```python
from build123d import *

# Parameters (mm, degrees)
CROQUIS1_R                   = 2.5
SALIENTE_EXTRUIR1_DEPTH      = 5
SALIENTE_EXTRUIR2_DEPTH      = 6
SALIENTE_EXTRUIR5_DEPTH      = 2
SALIENTE_EXTRUIR5_DEPTH_BACK = 0.1
CROQUIS2_W                   = 41.5
CROQUIS2_H                   = 5.75
CROQUIS2_H_2                 = 4
CROQUIS2_H_3                 = 1.75
CROQUIS2_W_2                 = 1.75
CROQUIS3_R                   = 2
SALIENTE_EXTRUIR6_DEPTH      = 8
CORTAR_EXTRUIR1_REACH        = 36.373
CORTAR_EXTRUIR2_START        = -3
CROQUIS4_R                   = 3.5
CROQUIS4_R_2                 = 2
CORTAR_EXTRUIR2_DEPTH        = 3
REDONDEO1_R                  = 2
REDONDEO2_R                  = 2


with BuildPart() as part:
    # Croquis1 → Saliente-Extruir1 (new body)
    with BuildSketch(Plane(origin=(0, 0, 0), x_dir=(1, 0, 0), z_dir=(0, 1, 0))):
        with BuildLine():
            Line((-22.5, -22.5), (22.5, -22.5))
            Line((22.5, -22.5), (22.5, -20.75))
            Line((22.5, -20.75), (-3.5, -20.75))
            ThreePointArc((-3.5, -20.75), (-7.5, -16.75), (-3.5, -12.75))
            Line((-3.5, -12.75), (22.5, -12.75))
            Line((22.5, -12.75), (22.5, 22.5))
            Line((22.5, 22.5), (-22.5, 22.5))
            Line((-22.5, 22.5), (-22.5, 20.75))
            Line((-22.5, 20.75), (3.5, 20.75))
            ThreePointArc((3.5, 20.75), (7.5, 16.75), (3.5, 12.75))
            Line((3.5, 12.75), (-22.5, 12.75))
            Line((-22.5, 12.75), (-22.5, -22.5))
        make_face()
        with Locations(Location((0, 0, 0), (0, 0, 270))):
            Circle(CROQUIS1_R, mode=Mode.SUBTRACT)
    extrude(amount=-SALIENTE_EXTRUIR1_DEPTH)

    # Croquis1<3> → Saliente-Extruir2 (add)
    with BuildSketch(Plane(origin=(0, 0, 0), x_dir=(1, 0, 0), z_dir=(0, 1, 0))):
        Polygon((-22.5, 7.75), (-22.5, -22.5), (22.5, -22.5), (22.5, -20.75), (-3.5, -20.75), (-20.75, -20.75), (-20.75, 7.75), align=None)
        Polygon((-22.5, 22.5), (-22.5, 20.75), (3.5, 20.75), (20.75, 20.75), (20.75, -7.75), (22.5, -7.75), (22.5, 22.5), align=None)
    extrude(amount=SALIENTE_EXTRUIR2_DEPTH)

    # Croquis2 → Saliente-Extruir5 (add, two sides: drawn at the far end of the back side and taken through both)
    with BuildSketch(Plane(origin=(0, 6, 0), x_dir=(1, 0, 0), z_dir=(0, 1, 0)).offset(-SALIENTE_EXTRUIR5_DEPTH_BACK)):
        with Locations((0, 19.625)):
            Rectangle(CROQUIS2_W, CROQUIS2_H)
        Polygon((-20.75, 22.5), (-22.5, 22.5), (-22.5, 7.75), (-20.75, 7.75), (-20.75, 16.75), align=None)
        with Locations((0, -18.75)):
            Rectangle(CROQUIS2_W, CROQUIS2_H_2)
        with Locations((0, -21.625)):
            Rectangle(CROQUIS2_W, CROQUIS2_H_3)
        Polygon((-20.75, 7.75), (-22.5, 7.75), (-22.5, -22.5), (-20.75, -22.5), (-20.75, -20.75), (-20.75, -16.75), align=None)
        Polygon((22.5, 22.5), (20.75, 22.5), (20.75, 16.75), (20.75, -16.75), (20.75, -20.75), (22.5, -20.75), align=None)
        with Locations((21.625, -21.625)):
            Rectangle(CROQUIS2_W_2, CROQUIS2_H_3)
    extrude(amount=SALIENTE_EXTRUIR5_DEPTH + SALIENTE_EXTRUIR5_DEPTH_BACK)

    # Croquis3 → Saliente-Extruir6 (add)
    with BuildSketch(Plane(origin=(0, 8, 0), x_dir=(1, 0, 0), z_dir=(0, 1, 0))):
        with BuildLine():
            Line((-20.75, 5), (-20.75, -5))
            Line((-20.75, -5), (-17.5, -5))
            Line((-17.5, -5), (-17.5, -2))
            ThreePointArc((-17.5, -2), (-19.5, 0), (-17.5, 2))
            Line((-17.5, 2), (-17.5, 5))
            Line((-17.5, 5), (-20.75, 5))
        make_face()
        with Locations((-17.5, 0)):
            Circle(CROQUIS3_R)
        with BuildLine():
            Line((-17.5, -5), (-17.5, 5))
            ThreePointArc((-17.5, 5), (-12.5, 0), (-17.5, -5))
        make_face()
        with BuildLine():
            ThreePointArc((-17.5, 2), (-19.5, 0), (-17.5, -2))
            Line((-17.5, -2), (-17.5, 2))
        make_face()
        with BuildLine():
            Line((-17.5, 2), (-17.5, -2))
            ThreePointArc((-17.5, -2), (-16.085786438, -1.414213562), (-15.5, 0))
            ThreePointArc((-15.5, 0), (-16.085786438, 1.414213562), (-17.5, 2))
        make_face()
    saliente_extruir6 = extrude(amount=-SALIENTE_EXTRUIR6_DEPTH)

    # Croquis3<3> → Cortar-Extruir1 (cut, up to next)
    with BuildSketch(Plane(origin=(0, 8, 0), x_dir=(1, 0, 0), z_dir=(0, 1, 0)), mode=Mode.PRIVATE) as cortar_extruir1_sk1:
        with BuildLine():
            ThreePointArc((-17.5, 2), (-19.5, 0), (-17.5, -2))
            Line((-17.5, -2), (-17.5, 2))
        make_face()
    cortar_extruir1_tool1 = extrude(cortar_extruir1_sk1.sketch, amount=-CORTAR_EXTRUIR1_REACH, mode=Mode.PRIVATE) & part.part
    # Croquis3<3> → Cortar-Extruir1 (cut, up to next)
    with BuildSketch(Plane(origin=(0, 8, 0), x_dir=(1, 0, 0), z_dir=(0, 1, 0)), mode=Mode.PRIVATE) as cortar_extruir1_sk2:
        with BuildLine():
            Line((-17.5, 2), (-17.5, -2))
            ThreePointArc((-17.5, -2), (-16.085786438, -1.414213562), (-15.5, 0))
            ThreePointArc((-15.5, 0), (-16.085786438, 1.414213562), (-17.5, 2))
        make_face()
    cortar_extruir1_tool2 = extrude(cortar_extruir1_sk2.sketch, amount=-CORTAR_EXTRUIR1_REACH, mode=Mode.PRIVATE) & part.part
    # Croquis3<3> → Cortar-Extruir1 (cut, up to next)
    with BuildSketch(Plane(origin=(0, 8, 0), x_dir=(1, 0, 0), z_dir=(0, 1, 0)), mode=Mode.PRIVATE) as cortar_extruir1_sk3:
        with BuildLine():
            ThreePointArc((-17.5, 2), (-19.5, 0), (-17.5, -2))
            Line((-17.5, -2), (-17.5, 2))
        make_face()
    cortar_extruir1_tool3 = extrude(cortar_extruir1_sk3.sketch, amount=-CORTAR_EXTRUIR1_REACH, mode=Mode.PRIVATE) & part.part
    # Croquis3<3> → Cortar-Extruir1 (cut, up to next)
    with BuildSketch(Plane(origin=(0, 8, 0), x_dir=(1, 0, 0), z_dir=(0, 1, 0)), mode=Mode.PRIVATE) as cortar_extruir1_sk4:
        with BuildLine():
            Line((-17.5, 2), (-17.5, -2))
            ThreePointArc((-17.5, -2), (-16.085786438, -1.414213562), (-15.5, 0))
            ThreePointArc((-15.5, 0), (-16.085786438, 1.414213562), (-17.5, 2))
        make_face()
    cortar_extruir1_tool4 = extrude(cortar_extruir1_sk4.sketch, amount=-CORTAR_EXTRUIR1_REACH, mode=Mode.PRIVATE) & part.part
    cortar_extruir1_1 = cortar_extruir1_tool1.solids().sort_by_distance((-18.348826, 8, 0))[0]
    add(cortar_extruir1_1, mode=Mode.SUBTRACT)
    cortar_extruir1_2 = cortar_extruir1_tool2.solids().sort_by_distance((-16.651174, 8, 0))[0]
    add(cortar_extruir1_2, mode=Mode.SUBTRACT)
    cortar_extruir1_3 = cortar_extruir1_tool3.solids().sort_by_distance((-18.348826, 8, 0))[0]
    add(cortar_extruir1_3, mode=Mode.SUBTRACT)
    cortar_extruir1_4 = cortar_extruir1_tool4.solids().sort_by_distance((-16.651174, 8, 0))[0]
    add(cortar_extruir1_4, mode=Mode.SUBTRACT)
    cortar_extruir1 = cortar_extruir1_1 + cortar_extruir1_2 + cortar_extruir1_3 + cortar_extruir1_4  # Cortar-Extruir1 as one shape, for the pattern or mirror that repeats it

    # Simetría1: Saliente-Extruir6, Cortar-Extruir1 across plane
    add(saliente_extruir6.mirror(Plane(origin=(0, 0, 0), x_dir=(0, 0, 1), z_dir=(1, 0, 0))))
    add(cortar_extruir1.mirror(Plane(origin=(0, 0, 0), x_dir=(0, 0, 1), z_dir=(1, 0, 0))), mode=Mode.SUBTRACT)

    # Croquis4 → Cortar-Extruir2 (cut)
    # profile 1 of 2: a face of its own
    with BuildSketch(Plane.XZ.offset(5).offset(CORTAR_EXTRUIR2_START)):
        with Locations(Location((-17.5, 0, 0), (0, 0, 270))):
            Circle(CROQUIS4_R)
        with Locations(Location((-17.5, 0, 0), (0, 0, 90))):
            Circle(CROQUIS4_R_2, mode=Mode.SUBTRACT)
    # profile 2 of 2: a face of its own
    with BuildSketch(Plane.XZ.offset(5).offset(CORTAR_EXTRUIR2_START)):
        with Locations(Location((17.5, 0, 0), (0, 0, 270))):
            Circle(CROQUIS4_R)
        with Locations(Location((17.5, 0, 0), (0, 0, 90))):
            Circle(CROQUIS4_R_2, mode=Mode.SUBTRACT)
    extrude(amount=CORTAR_EXTRUIR2_DEPTH, mode=Mode.SUBTRACT)

    # Redondeo1
    redondeo1_edges = [part.edges().sort_by_distance(p)[0] for p in [
        (20.75, 6.95, 16.75),
        (-20.75, 6.95, 16.75),
        (20.75, 6.95, -16.75),
        (-20.75, 4, -5),
        (-20.75, 4, 5),
        (20.75, 4, 5),
        (20.75, 4, -5),
        (-20.75, 6.95, -16.75),
    ]]
    fillet(redondeo1_edges, radius=REDONDEO1_R)

    # Redondeo2
    redondeo2_edges = [part.edges().sort_by_distance(p)[0] for p in [
        (-22.5, 1.5, -22.5),
        (22.5, 1.5, -22.5),
        (-22.5, 1.5, 22.5),
        (22.5, 1.5, 22.5),
        (20.75, 2.95, -20.75),
        (-20.75, 2.95, 20.75),
    ]]
    fillet(redondeo2_edges, radius=REDONDEO2_R)


solid = part.part
```
Geometry check sheet. Reference: the model listing, model coordinates, mm. A direction names the side the tool comes from. Round coordinates to 2 decimals unless told otherwise and drop trailing zeros. Loops run counter-clockwise (first coordinate to the right, second up) from the corner with the lowest first, then second, coordinate; pieces in that order, holes last. Notation, with made-up numbers: (0, 57) -> (44, 57) arc R23 cw to (44, 94) -> close; hole circle Ø5 at (88, -23.5). An arc over 180 degrees is marked (long way). Use a Markdown table: item, result.
(1) Mould release check, pull along Z, two halves, no side actions. Record for faces 4 (the flat face through (0, -5, 5)), 5 (the cylindrical face through (7.5, -2.5, -16.8)), 6 (the cylindrical face through (21.9, 1.59, -21.93)): released by +Z, released by -Z, zero draft, split by the parting line, or undercut.
Calculated:
| item | result |
|---|---|
| face 4 | zero draft |
| face 5 | undercut |
| face 6 | released by -Z |
(2) Sectioned sample at C-C (x = -9). Enter the section's corners in (y, z).
Calculated:
| item | result |
|---|---|
| outline | (-5, -22.5) -> (8, -22.5) -> (8, -16.75) -> (5.9, -16.75) -> (5.9, -20.75) -> (-5, -20.75) -> close; (-5, -12.75) -> (0, -12.75) -> (0, 20.75) -> (5.9, 20.75) -> (5.9, 16.75) -> (8, 16.75) -> (8, 22.5) -> (-5, 22.5) -> close |
(3) Go/stop test with flat-tipped pins: P1, Ø6.5, axis at y = 5.5, z = 15.5, coming from the +X side; P2, Ø4, axis at x = -11.5, z = 14.5, coming from the +Y side; P3, Ø0.9, axis at x = -21.5, y = 2.5, coming from the -Z side; P4, Ø1, axis at y = 4.5, z = -15.5, coming from the -X side. Record where each tip stops, or that it passes through.
Calculated:
| item | result |
|---|---|
| P1 | x = 22.5 |
| P2 | y = 0 |
| P3 | z = -22.42 |
| P4 | x = 20.75 |
(4) Sectioned sample at D-D (x = 0). Enter the section's corners in (y, z), then the cut area to 3 significant figures.
Calculated:
| item | result |
|---|---|
| outline | (-5, -22.5) -> (8, -22.5) -> (8, -16.75) -> (5.9, -16.75) -> (5.9, -20.75) -> (-5, -20.75) -> close; (-5, -12.75) -> (0, -12.75) -> (0, -2.5) -> (-5, -2.5) -> close; (-5, 2.5) -> (0, 2.5) -> (0, 12.75) -> (-5, 12.75) -> close; (-5, 20.75) -> (5.9, 20.75) -> (5.9, 16.75) -> (8, 16.75) -> (8, 22.5) -> (-5, 22.5) -> close |
| area | 165 mm² |
(5) Set-up check for faces 1 (the flat face through (-7, 0, -20.75)), 2 (the flat face through (-19, -2, -2)), 3 (the flat face through (-18, 4, 5)): record each of +Z, -Z, +X, -X, +Y, -Y from which the full face is reachable in a straight line by a thin tool's end or side.
Calculated:
| item | result |
|---|---|
| face 1 | -X |
| face 2 | -Y |
| face 3 | +Y |
(6) Sectioned sample at B-B (z = 11). Enter the section's corners in (x, y), then the cut area to 3 significant figures.
Calculated:
| item | result |
|---|---|
| outline | (-22.5, -5) -> (22.5, -5) -> (22.5, 0) -> (-20.75, 0) -> (-20.75, 8) -> (-22.5, 8) -> close; (20.75, 5.9) -> (22.5, 5.9) -> (22.5, 8) -> (20.75, 8) -> close |
| area | 243 mm² |
(7) Sectioned sample at A-A (y = 1.75). Give the number of separate pieces and of enclosed holes in the cut face, then the cut area to 3 significant figures.
Calculated:
| item | result |
|---|---|
| separate pieces | 2 |
| enclosed holes | 2 |
| area | 377 mm² |
(8) Scan lines: probe 1 along X at (y, z) = (-2.95, 0); probe 2 along Z at (x, y) = (14.5, 6); probe 3 along Z at (x, y) = (13.5, 7.5). Record each from-to range of solid material in increasing order.
Calculated:
| item | result |
|---|---|
| probe 1 | -22.5 to -21, -14 to -2.5, 2.5 to 14, 21 to 22.5 |
| probe 2 | -22.5 to -16.75, -4 to 4, 16.75 to 22.5 |
| probe 3 | -22.5 to -16.75, -3 to 3, 16.75 to 22.5 |
